Answer from the drawing. Dimensions are ordinates in mm from the lowest x, y and z of the part. A direction names the side the tool comes from. Give positions to 0.01 mm unless a question says otherwise; leave off trailing zeros. Write each loop counter-clockwise with the first axis right and the second up, starting at its lowest first coordinate (ties: lowest second). Pieces come first, ordered by that corner, then holes. Notation, with made-up numbers: M 10.25,-3 L 34.25,-3 A5 ccw 34.25,6 Z; hole C 74,74 d2. An arc over 180 degrees is marked long. Answer as a JSON object with one key per item and string values.
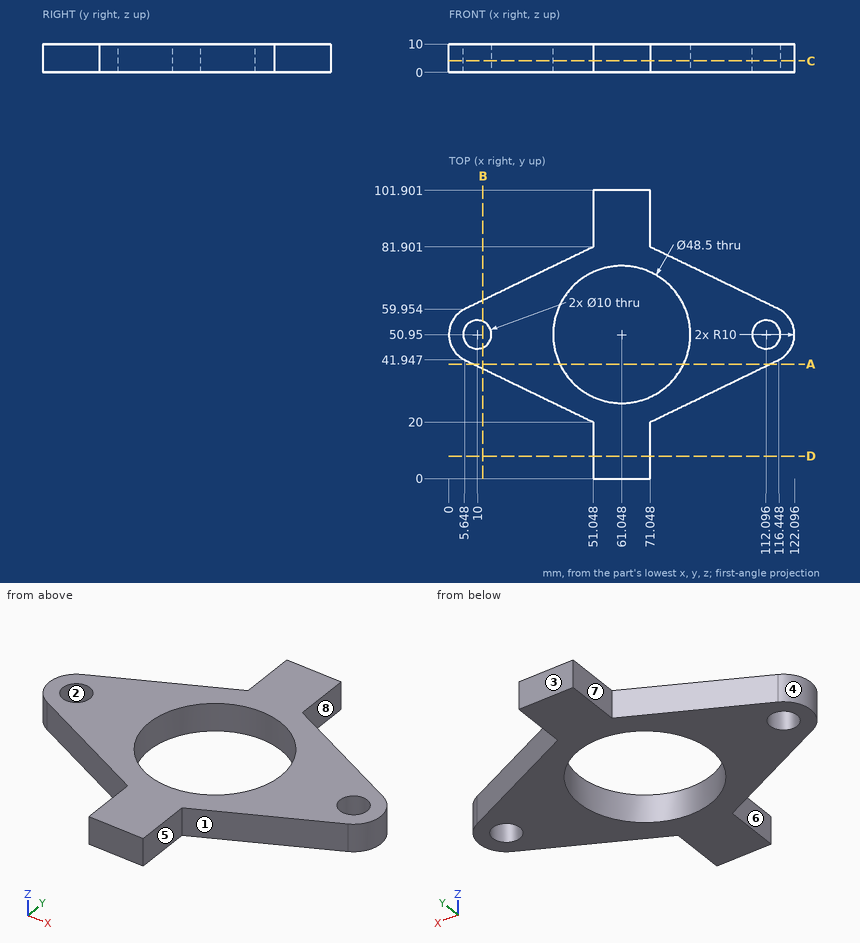
1. Consider line 1 along X through (y, z) = (9, 1.5); line 2 along Y through (x, z) = (68, 8.5); line 3 along X through (y, z) = (73.5, 7) (1 decimal). Determine where each line is inside the solid, lowest interval first.
Verdict:
{"line 1": "x = 51.05 to 71.05", "line 2": "y = 0 to 27.72, 74.18 to 101.9", "line 3": "x = 33.7 to 52.1, 70 to 88.4"}
2. A cutting plane is placed at D-D, the plane y = 8. Give the vertices of the cut face in (x, z).
Verdict:
{"outline": "M 51.05,0 L 71.05,0 L 71.05,10 L 51.05,10 Z"}
3. A cutting plane is placed at C-C, the plane z = 4. Count the separate pieces of the cut face and the enclosed holes in it, plus the area to 3 significant figures.
Verdict:
{"separate pieces": "1", "enclosed holes": "3", "area": "3,810 mm2"}
4. Flat-ended cylindrical pins translate along their axes: pin 1 (1 mm diameter, centred on y = 17.5, z = 1.5, fed in from -X); pin 2 (1.5 mm diameter, centred on y = 79.5, z = 2.5, fed in from +X) (1 decimal); pin 3 (5 mm diameter, centred on y = 5.5, z = 7.5, fed in from +X). Find the tip coordinate at first contact, or state that the pin passes through.
Verdict:
{"pin 1": "stops at x = 51.05", "pin 2": "stops at x = 77.6", "pin 3": "stops at x = 71.05"}
5. For the marked faces 4, 5, 6, 7 and 8, determine the directions among +Z, -Z, +X, -X, +Y, -Y from which every point of the face is accessible in a straight line to the end or side of a thin tool.
Verdict:
{"face 4": "+Z, -Z, -X", "face 5": "+Z, -Z, +X, -Y", "face 6": "+Z, -Z, -X, -Y", "face 7": "+Z, -Z, -X, +Y", "face 8": "+Z, -Z, +X, +Y"}
6. The mould has two halves that part along X. Classify the marked faces 1, 2 and 3: released by +X, released by -X, zero draft, split by the parting line, or undercut.
Verdict:
{"face 1": "released by +X", "face 2": "undercut", "face 3": "zero draft"}
7. A cutting plane is placed at B-B, the plane x = 12. Give the vertices of the cut face in (y, z) (1 decimal), plus the area to 3 significant figures.
Verdict:
{"outline": "M 38.9,0 L 46.4,0 L 46.4,10 L 38.9,10 Z; M 55.5,0 L 63,0 L 63,10 L 55.5,10 Z", "area": "150 mm2"}
8. A cutting plane is placed at A-A, the plane y = 40.5. Give the vertices of the cut face in (x, z) (1 decimal).
Verdict:
{"outline": "M 8.6,0 L 39.2,0 L 39.2,10 L 8.6,10 Z; M 82.9,0 L 113.5,0 L 113.5,10 L 82.9,10 Z"}
